```python
from build123d import *

# Parameters (mm, degrees)
SKETCH_1_R          = 4
EXTRUDE_1_DEPTH     = 30
SKETCH_3_R          = 2
CUT_EXTRUDE_1_DEPTH = 100


with BuildPart() as part:
    # 草图1 → 凸台-拉伸1 (new body)
    with BuildSketch(Plane(origin=(0, 0, 0), x_dir=(1, 0, 0), z_dir=(0, 1, 0))):
        with BuildLine():
            Line((-40.566755923, 0.414213562), (-31.980969486, 0.414213562))
            ThreePointArc((-31.980969486, 0.414213562), (-31.598286053, 0.49033403), (-31.273862704, 0.707106781))
            Line((-31.273862704, 0.707106781), (-31.152542361, 0.828427125))
            ThreePointArc((-31.152542361, 0.828427125), (-30.828119012, 1.045199876), (-30.44543558, 1.121320344))
            Line((-30.44543558, 1.121320344), (-18.761824504, 1.121320344))
            ThreePointArc((-18.761824504, 1.121320344), (-18.379141072, 1.045199876), (-18.054717723, 0.828427125))
            Line((-18.054717723, 0.828427125), (-17.933397379, 0.707106781))
            ThreePointArc((-17.933397379, 0.707106781), (-17.60897403, 0.49033403), (-17.226290598, 0.414213562))
            Line((-17.226290598, 0.414213562), (-8.64050416, 0.414213562))
            ThreePointArc((-8.64050416, 0.414213562), (-7.933397379, 0.707106781), (-7.64050416, 1.414213562))
            Line((-7.64050416, 1.414213562), (-7.64050416, 6))
            ThreePointArc((-7.64050416, 6), (-7.716624628, 6.382683432), (-7.933397379, 6.707106781))
            Line((-7.933397379, 6.707106781), (-8.761824504, 7.535533906))
            ThreePointArc((-8.761824504, 7.535533906), (-8.978597255, 7.859957255), (-9.054717723, 8.242640687))
            Line((-9.054717723, 8.242640687), (-9.054717723, 16.828427125))
            ThreePointArc((-9.054717723, 16.828427125), (-9.347610942, 17.535533906), (-10.054717723, 17.828427125))
            Line((-10.054717723, 17.828427125), (-15.64050416, 17.828427125))
            ThreePointArc((-15.64050416, 17.828427125), (-16.023187593, 17.904547592), (-16.347610942, 18.121320344))
            Line((-16.347610942, 18.121320344), (-19.29735841, 21.071067812))
            ThreePointArc((-19.29735841, 21.071067812), (-19.621781759, 21.287840563), (-20.004465191, 21.363961031))
            Line((-20.004465191, 21.363961031), (-29.202794893, 21.363961031))
            ThreePointArc((-29.202794893, 21.363961031), (-29.585478325, 21.287840563), (-29.909901674, 21.071067812))
            Line((-29.909901674, 21.071067812), (-32.859649142, 18.121320344))
            ThreePointArc((-32.859649142, 18.121320344), (-33.184072491, 17.904547592), (-33.566755923, 17.828427125))
            Line((-33.566755923, 17.828427125), (-39.152542361, 17.828427125))
            ThreePointArc((-39.152542361, 17.828427125), (-39.859649142, 17.535533906), (-40.152542361, 16.828427125))
            Line((-40.152542361, 16.828427125), (-40.152542361, 8.242640687))
            ThreePointArc((-40.152542361, 8.242640687), (-40.228662828, 7.859957255), (-40.44543558, 7.535533906))
            Line((-40.44543558, 7.535533906), (-41.273862704, 6.707106781))
            ThreePointArc((-41.273862704, 6.707106781), (-41.490635456, 6.382683432), (-41.566755923, 6))
            Line((-41.566755923, 6), (-41.566755923, 1.414213562))
            ThreePointArc((-41.566755923, 1.414213562), (-41.273862704, 0.707106781), (-40.566755923, 0.414213562))
        make_face()
        with Locations(Location((-24.603630042, 11.242640687, 0), (0, 0, 270))):
            Circle(SKETCH_1_R, mode=Mode.SUBTRACT)
    extrude(amount=EXTRUDE_1_DEPTH)

    # 草图3 → 切除-拉伸1 (cut)
    with BuildSketch(Plane.XY.offset(-0.414213562)):
        with Locations((-12.603630042, 6)):
            Circle(SKETCH_3_R)
        with Locations((-36.603630042, 6)):
            Circle(SKETCH_3_R)
        with Locations((-36.603630042, 24)):
            Circle(SKETCH_3_R)
        with Locations((-12.603630042, 24)):
            Circle(SKETCH_3_R)
    extrude(amount=-CUT_EXTRUDE_1_DEPTH, mode=Mode.SUBTRACT)


solid = part.part
```
Design review of the part built by this model. Coordinates are the model's own, in mm. A direction names the side the tool comes from. Coordinates: 2 decimals unless noted, no trailing zeros. Write each loop counter-clockwise with the first axis right and the second up, starting at its lowest first coordinate (ties: lowest second). Pieces come first, ordered by that corner, then holes.
1) Add section B-B (y = 24.5). State how many separate pieces and enclosed holes the cut face has, plus the area to 3 significant figures.
2) Add section A-A (z = -4). Write out the cut boundary in (x, y).
3) Add section D-D (z = -17.25). Write out the cut boundary in (x, y), plus the area to 3 significant figures.
4) Insertion check: pin 1 (7 mm diameter, centred on y = 11.5, z = -11.5, fed in from -X); pin 2 (1.7 mm diameter, centred on x = -37.5, y = 9, fed in from -Z); pin 3 (7 mm diameter, centred on y = 18.5, z = -13.5, fed in from +X); pin 4 (6.5 mm diameter, centred on x = -24.6, z = -11.24, fed in from -Y). Each pin has a flat end and moves straight along its axis. Give the tip position at first contact, or say it passes through.
5) Mouldability with a two-part tool opening along Z and no side actions: class faces 1 (the cylindrical face through (-7.94, 14.79, -0.7)), 2 (the cylindrical face through (-28.51, 14.79, -12.11)), 3 (the flat face through (-7.641, 15, -4)), 4 (the cylindrical face through (-39.852, 14.79, -17.543)) as +Z half, -Z half, draft (parallel to the pull), parting line (faces both ways), or undercut.
6) Machinability: for faces 5 (the cylindrical face through (-14.19, 22.78, -9)), 6 (the flat face through (-13, 15, -17.828)), 7 (the flat face through (-25, 15, -1.121)), which of the approach directions +Z, -Z, +X, -X, +Y, -Y give a long, thin tool a straight path to every point of the face, cutting with its end or side? Answer none if there is none.
7) To check wall thickness, follow L1, parallel to Y at x = -38, z = -14.25; L2, parallel to X at y = 22.75, z = -12.25; L3, parallel to X at y = 22.5, z = -11.5. State the ranges of each line that lie inside material, in increasing order.
Check result:
1. separate pieces: 3
1. enclosed holes: 1
1. area: 413 mm2
2. outline: (-41.57, 0) - (-7.64, 0) - (-7.64, 30) - (-41.57, 30) - close; hole circle Ø4 at (-36.6, 6); hole circle Ø4 at (-36.6, 24); hole circle Ø4 at (-12.6, 6); hole circle Ø4 at (-12.6, 24)
3. outline: (-40.06, 0) - (-9.15, 0) - (-9.15, 30) - (-40.06, 30) - close; hole circle Ø4 at (-36.6, 6); hole circle Ø4 at (-36.6, 24); hole circle Ø4 at (-12.6, 6); hole circle Ø4 at (-12.6, 24)
3. area: 877 mm2
4. pin 1: stops at x = -40.18
4. pin 2: stops at z = -17.83
4. pin 3: stops at x = -9.05
4. pin 4: passes through
5. face 1: +Z half
5. face 2: undercut
5. face 3: draft
5. face 4: -Z half
6. face 5: +Z, -Z
6. face 6: -Z, +X, +Y, -Y
6. face 7: +Z, +Y, -Y
7. L1: y = 0 to 4.57, 7.43 to 22.57, 25.43 to 30
7. L2: x = -40.15 to -38.16, -35.04 to -28.47, -20.73 to -14.16, -11.04 to -9.05
7. L3: x = -40.15 to -37.93, -35.28 to -28.6, -20.61 to -13.93, -11.28 to -9.05
